Geometry check sheet. Reference: the model listing, model coordinates, mm. Round coordinates to 2 decimals unless told otherwise and drop trailing zeros. Order: outer loops, then holes, each group sorted by start corner. A loop starts at its lowest first (then second) coordinate and runs counter-clockwise, first axis right, second up.
(1) Gauge pin test, flat ends, axial feed: P1, Ø3, axis at x = 215, z = 40, coming from the -Y side; P2, Ø5, axis at x = 169, y = 34, coming from the -Z side; P3, Ø12, axis at x = 184, y = -21.5, coming from the +Z side. Record the tip position at first contact, or that the pin passes through.
(2) Thickness scan on L1, parallel to Y at x = 65, z = 34.5; L2, parallel to Z at x = 154, y = -40; L3, parallel to Z at x = 261, y = 26. Record the ranges inside material, lowest first.
(3) Cross-section at B-B on y = 15. Enter the section's corners in (x, z), and give its area (3 significant figures).
(4) Cross-section at A-A on x = 140.5. Enter the section's corners in (y, z).
(5) Cross-section at C-C on z = -36. Enter the section's corners in (x, y), and give its area (3 significant figures).
from build123d import *

# Parameters (mm, degrees)
F1_DEPTH = 304.8


with BuildPart() as f1:
    # F0 (on Right) → F1 (new body)
    with BuildSketch(Plane.YZ):
        with BuildLine():
            Line((48.2470816248, -15.901544412), (-48.2470816248, 15.901544412))
            ThreePointArc((-48.2470816248, 15.901544412), (-15.901544412, -48.2470816248), (48.2470816248, -15.901544412))
        make_face()
        with BuildLine():
            ThreePointArc((48.2470816248, -15.901544412), (50.1577100082, -8.052585096), (50.8, 0))
            ThreePointArc((50.8, 0), (8.052585096, 50.1577100082), (-48.2470816248, 15.901544412))
            Line((-48.2470816248, 15.901544412), (48.2470816248, -15.901544412))
        make_face()
    extrude(amount=F1_DEPTH)


with BuildPart() as f2_1:
    # F2: copy of F1
    add(f1.part)


solid = f1.part
Found:
1. P1: stops at y = -33.14
1. P2: stops at z = -39.85
1. P3: stops at z = 48.38
2. L1: y = -37.29 to 37.29
2. L2: z = -31.32 to 31.32
2. L3: z = -43.64 to 43.64
3. outline: (0, -48.53) - (304.8, -48.53) - (304.8, 48.53) - (0, 48.53) - close
3. area: 29,600 mm2
4. outline: circle Ø101.6 at (0, 0)
5. outline: (0, -35.84) - (304.8, -35.84) - (304.8, 35.84) - (0, 35.84) - close
5. area: 21,800 mm2
